Part model, mm, in its own coordinate system. Face numbers are marked on the shaded views. A direction names the side the tool comes from. Give positions to 0.01 mm unless a question says otherwise; leave off trailing zeros. Write each loop counter-clockwise with the first axis right and the second up, starting at its lowest first coordinate (ties: lowest second). Pieces come first, ordered by that corner, then holes. Notation, with made-up numbers: (6.5, 47) - (36.5, 47) arc R20 ccw to (36.5, 67) - close; hole circle Ø11 at (-9, 38). An arc over 180 degrees is marked (long way). Answer in a Markdown table with one row per item. Add a question column.
1. Band-saw the part on A-A on x = 1.5. Write the cut outline in (y, z), plus the area to 3 significant figures.
2. Band-saw the part on B-B on y = 1.75. Write the cut outline in (x, z).
3. Drop flat-ended pins along their axis: pin 1 Ø3 at (x, z) = (10.5, 0.5) entering from +Y; pin 2 Ø3 at (x, y) = (17, -2) entering from +Z; pin 3 Ø0.7 at (y, z) = (-1, 0) entering from -X. Give the stop position or say it passes through.
4. Pull direction Z, two halves, no side cores. Call the marked faces 3, 4, 5 and 6: released by +Z, released by -Z, zero draft, split by the parting line, or undercut.
5. Band-saw the part on C-C on y = 3.25. Write the cut outline in (x, z), plus the area to 3 significant figures.
6. Probe line 1 along Z through (x, y) = (16, -1.75); line 2 along Y through (x, z) = (12, 2.5); line 3 along Y through (x, z) = (17.25, -0.3). List the from-to ranges inside material, lowest first.
7. Band-saw the part on D-D on x = 17.25. Write the cut outline in (y, z).
8. Which spindle directions (+Z, -Z, +X, -X, +Y, -Y) get a long thin tool onto all of the face, cutting with end or side? Do the marked faces 1 and 2. Say none if no direction does.
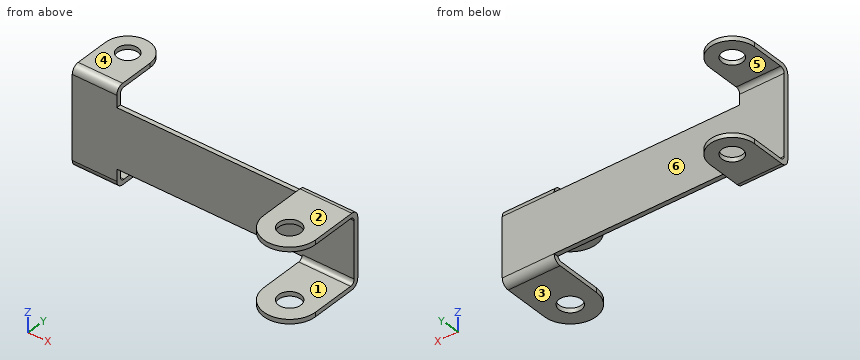
```python
from build123d import *

# Parameters (mm, degrees)
SKETCH1_W           = 19
SKETCH1_H           = 4
BOSS_EXTRUDE1_DEPTH = 0.3
SKETCH2_W           = 3
SKETCH2_H           = 1.3
BOSS_EXTRUDE2_DEPTH = 0.3
SKETCH3_W           = 3
SKETCH3_H           = 0.3
BOSS_EXTRUDE3_DEPTH = 4
FILLET1_RADIUS      = 1.5
FILLET1_LENGTH      = 0.3
FILLET2_RADIUS      = 1.5
FILLET2_LENGTH      = 0.3
SKETCH4_R           = 0.7
CUT_EXTRUDE1_DEPTH  = 21.568179307
SKETCH6_W           = 3.5
SKETCH6_H           = 0.5
BOSS_EXTRUDE4_DEPTH = 0.3
SKETCH7_W           = 3.5
SKETCH7_H           = 0.3
BOSS_EXTRUDE5_DEPTH = 5
FILLET3_RADIUS      = 1.75
FILLET3_LENGTH      = 0.3
FILLET4_RADIUS      = 1.75
FILLET4_LENGTH      = 0.3
SKETCH8_R           = 0.75
CUT_EXTRUDE2_DEPTH  = 21.485116548
FILLET5_R           = 0.3
FILLET6_R           = 0.5


with BuildPart() as part:
    # Sketch1 → Boss-Extrude1 (new body)
    with BuildSketch(Plane(origin=(0, 0, 0), x_dir=(1, 0, 0), z_dir=(0, 1, 0))):
        with Locations((9.5, -2)):
            Rectangle(SKETCH1_W, SKETCH1_H)
    extrude(amount=BOSS_EXTRUDE1_DEPTH)

    # Sketch2 → Boss-Extrude2 (add)
    with BuildSketch(Plane.XZ):
        with Locations((1.5, -0.65)):
            Rectangle(SKETCH2_W, SKETCH2_H)
        with Locations((1.5, 4.65)):
            Rectangle(SKETCH2_W, SKETCH2_H)
    extrude(amount=-BOSS_EXTRUDE2_DEPTH)

    # Sketch3 → Boss-Extrude3 (add)
    with BuildSketch(Plane(origin=(0, 0.3, 0), x_dir=(1, 0, 0), z_dir=(0, 1, 0))):
        with Locations((1.5, 1.15)):
            Rectangle(SKETCH3_W, SKETCH3_H)
        with Locations((1.5, -5.15)):
            Rectangle(SKETCH3_W, SKETCH3_H)
    extrude(amount=BOSS_EXTRUDE3_DEPTH)

    # Fillet1: full round fillet: the end face becomes a half cylinder, R = half its width
    fillet1_face = Plane((1.5, 4.3, -1.15), x_dir=(0, 0, 1), z_dir=(0, 1, 0))  # on the end face: x along it, z out of the body
    fillet1_slab = fillet1_face.offset(-FILLET1_RADIUS / 2) * Box(FILLET1_LENGTH, 2 * FILLET1_RADIUS, FILLET1_RADIUS, mode=Mode.PRIVATE)  # the body's end, R deep
    fillet1_round = Plane((1.5, 2.8, -1.15), x_dir=(0, 1, 0), z_dir=(0, 0, 1)) * Cylinder(FILLET1_RADIUS, FILLET1_LENGTH, mode=Mode.PRIVATE)  # its axis R under the face
    add(fillet1_slab - fillet1_round, mode=Mode.SUBTRACT)

    # Fillet2: full round fillet: the end face becomes a half cylinder, R = half its width
    fillet2_face = Plane((1.5, 4.3, 5.15), x_dir=(0, 0, -1), z_dir=(0, 1, 0))  # on the end face: x along it, z out of the body
    fillet2_slab = fillet2_face.offset(-FILLET2_RADIUS / 2) * Box(FILLET2_LENGTH, 2 * FILLET2_RADIUS, FILLET2_RADIUS, mode=Mode.PRIVATE)  # the body's end, R deep
    fillet2_round = Plane((1.5, 2.8, 5.15), x_dir=(0, 1, 0), z_dir=(0, 0, -1)) * Cylinder(FILLET2_RADIUS, FILLET2_LENGTH, mode=Mode.PRIVATE)  # its axis R under the face
    add(fillet2_slab - fillet2_round, mode=Mode.SUBTRACT)

    # Sketch4 → Cut-Extrude1 (cut, through all)
    with BuildSketch(Plane(origin=(0, 0, -1.3), x_dir=(-1, 0, 0), z_dir=(0, 0, -1))):
        with Locations((-1.5, 2.8)):
            Circle(SKETCH4_R)
    extrude(amount=-CUT_EXTRUDE1_DEPTH, mode=Mode.SUBTRACT)

    # Sketch6 → Boss-Extrude4 (add)
    with BuildSketch(Plane(origin=(0, 0.3, 0), x_dir=(1, 0, 0), z_dir=(0, 1, 0))):
        with Locations((17.25, 0.25)):
            Rectangle(SKETCH6_W, SKETCH6_H)
        with Locations((17.25, -4.25)):
            Rectangle(SKETCH6_W, SKETCH6_H)
    extrude(amount=-BOSS_EXTRUDE4_DEPTH)

    # Sketch7 → Boss-Extrude5 (add)
    with BuildSketch(Plane.XZ):
        with Locations((17.25, -0.35)):
            Rectangle(SKETCH7_W, SKETCH7_H)
        with Locations((17.25, 4.35)):
            Rectangle(SKETCH7_W, SKETCH7_H)
    extrude(amount=BOSS_EXTRUDE5_DEPTH)

    # Fillet3: full round fillet: the end face becomes a half cylinder, R = half its width
    fillet3_face = Plane((17.25, -5, 4.35), x_dir=(0, 0, -1), z_dir=(0, -1, 0))  # on the end face: x along it, z out of the body
    fillet3_slab = fillet3_face.offset(-FILLET3_RADIUS / 2) * Box(FILLET3_LENGTH, 2 * FILLET3_RADIUS, FILLET3_RADIUS, mode=Mode.PRIVATE)  # the body's end, R deep
    fillet3_round = Plane((17.25, -3.25, 4.35), x_dir=(0, -1, 0), z_dir=(0, 0, -1)) * Cylinder(FILLET3_RADIUS, FILLET3_LENGTH, mode=Mode.PRIVATE)  # its axis R under the face
    add(fillet3_slab - fillet3_round, mode=Mode.SUBTRACT)

    # Fillet4: full round fillet: the end face becomes a half cylinder, R = half its width
    fillet4_face = Plane((17.25, -5, -0.35), x_dir=(0, 0, -1), z_dir=(0, -1, 0))  # on the end face: x along it, z out of the body
    fillet4_slab = fillet4_face.offset(-FILLET4_RADIUS / 2) * Box(FILLET4_LENGTH, 2 * FILLET4_RADIUS, FILLET4_RADIUS, mode=Mode.PRIVATE)  # the body's end, R deep
    fillet4_round = Plane((17.25, -3.25, -0.35), x_dir=(0, -1, 0), z_dir=(0, 0, -1)) * Cylinder(FILLET4_RADIUS, FILLET4_LENGTH, mode=Mode.PRIVATE)  # its axis R under the face
    add(fillet4_slab - fillet4_round, mode=Mode.SUBTRACT)

    # Sketch8 → Cut-Extrude2 (cut, through all)
    with BuildSketch(Plane.XY.offset(4.5)):
        with Locations((17.25, -3.25)):
            Circle(SKETCH8_R)
    extrude(amount=-CUT_EXTRUDE2_DEPTH, mode=Mode.SUBTRACT)

    # Fillet5
    # the kernel refuses this fillet: 0.3 mm, written as the material it adds along each edge
    with BuildSketch(Plane(origin=(19, 0, -0.2), x_dir=(0, 0, 1), z_dir=(-1, 0, 0))) as fillet5_piece_1:
        with BuildLine():
            CenterArc((FILLET5_R, -FILLET5_R), FILLET5_R, 90, 90)
            Line((0, -FILLET5_R), (0, 0))
            Line((0, 0), (FILLET5_R, 0))
        make_face()
    extrude(amount=3.5)
    with BuildSketch(Plane(origin=(19, 0, 4.2), x_dir=(0, 0, -1), z_dir=(-1, 0, 0))) as fillet5_piece_2:
        with BuildLine():
            CenterArc((FILLET5_R, FILLET5_R), FILLET5_R, 180, 90)
            Line((0, FILLET5_R), (0, 0))
            Line((0, 0), (FILLET5_R, 0))
        make_face()
    extrude(amount=3.5)
    with BuildSketch(Plane(origin=(3, 0.3, -1), x_dir=(0, 0, 1), z_dir=(-1, 0, 0)), Plane(origin=(0, 0.3, 5), x_dir=(0, 0, -1), z_dir=(1, 0, 0))) as fillet5_piece_3:
        with BuildLine():
            CenterArc((FILLET5_R, FILLET5_R), FILLET5_R, 180, 90)
            Line((0, FILLET5_R), (0, 0))
            Line((0, 0), (FILLET5_R, 0))
        make_face()
    extrude(amount=3)

    # Fillet6
    fillet6_edges = [part.edges().sort_by_distance(p)[0] for p in [
        (1.5, 0, 5.3),
        (1.5, 0, -1.3),
        (17.25, 0.3, 4.5),
        (17.25, 0.3, -0.5),
    ]]
    fillet(fillet6_edges, radius=FILLET6_R)


solid = part.part
```
Values:
| question | item | result |
|---|---|---|
| 1 | outline | (0, -0.8) arc R0.5 ccw to (0.5, -1.3) - (2.1, -1.3) - (2.1, -1) - (0.6, -1) arc R0.3 cw to (0.3, -0.7) - (0.3, 4.7) arc R0.3 cw to (0.6, 5) - (2.1, 5) - (2.1, 5.3) - (0.5, 5.3) arc R0.5 ccw to (0, 4.8) - close; (3.5, -1.3) - (4.3, -1.3) - (4.3, -1) - (3.5, -1) - close; (3.5, 5) - (4.3, 5) - (4.3, 5.3) - (3.5, 5.3) - close |
| 1 | area | 3.47 mm² |
| 2 | outline | (0, -1.3) - (3, -1.3) - (3, -1) - (0, -1) - close; (0, 5) - (3, 5) - (3, 5.3) - (0, 5.3) - close |
| 3 | pin 1 | stops at y = 0.3 |
| 3 | pin 2 | stops at z = 4.5 |
| 3 | pin 3 | stops at x = 15.5 |
| 4 | face 3 | released by -Z |
| 4 | face 4 | released by +Z |
| 4 | face 5 | undercut |
| 4 | face 6 | undercut |
| 5 | outline | (0.07, -1.3) - (0.96, -1.3) - (0.96, -1) - (0.07, -1) - close; (0.07, 5) - (0.96, 5) - (0.96, 5.3) - (0.07, 5.3) - close; (2.04, -1.3) - (2.93, -1.3) - (2.93, -1) - (2.04, -1) - close; (2.04, 5) - (2.93, 5) - (2.93, 5.3) - (2.04, 5.3) - close |
| 5 | area | 1.07 mm² |
| 6 | line 1 | z = -0.5 to -0.2, 4.2 to 4.5 |
| 6 | line 2 | y = 0 to 0.3 |
| 6 | line 3 | y = -5 to -4, -2.5 to 0.2 |
| 7 | outline | (-5, -0.5) - (-4, -0.5) - (-4, -0.2) - (-5, -0.2) - close; (-5, 4.2) - (-4, 4.2) - (-4, 4.5) - (-5, 4.5) - close; (-2.5, -0.5) - (-0.2, -0.5) arc R0.5 ccw to (0.3, 0) - (0.3, 4) arc R0.5 ccw to (-0.2, 4.5) - (-2.5, 4.5) - (-2.5, 4.2) - (-0.3, 4.2) arc R0.3 cw to (0, 3.9) - (0, 0.1) arc R0.3 cw to (-0.3, -0.2) - (-2.5, -0.2) - close |
| 8 | face 1 | +X, -X, -Y |
| 8 | face 2 | +Z, +X, -X, +Y, -Y |
